```python
from build123d import *

# Parameters (mm, degrees)
ESBO_O1_R                = 1.5
RESSALTO_EXTRUS_O1_DEPTH = 1
ESBO_O2_W                = 25
ESBO_O2_H                = 1
RESSALTO_EXTRUS_O2_DEPTH = 5
ESBO_O3_R                = 1.75
CORTE_EXTRUS_O1_DEPTH    = 5
ESBO_O4_W                = 4.5
ESBO_O4_H                = 1
RESSALTO_EXTRUS_O3_DEPTH = 1.1
ESBO_O5_W                = 4.5
ESBO_O5_H                = 6.5
RESSALTO_EXTRUS_O4_DEPTH = 1


with BuildPart() as part:
    # Esboço1 → Ressalto-extrusão1 (new body)
    with BuildSketch(Plane.XY):
        Polygon((-2.930659551, 5.581459362), (-2.930659551, -2.668540638), (22.069340449, -2.668540638), (22.069340449, 5.581459362), (17.319340449, 5.581459362), (17.319340449, -1.668540638), (1.819340449, -1.668540638), (1.819340449, 5.581459362), align=None)
        with Locations((-0.180659551, 2.831459362)):
            Circle(ESBO_O1_R, mode=Mode.SUBTRACT)
        with Locations((19.319340449, 2.831459362)):
            Circle(ESBO_O1_R, mode=Mode.SUBTRACT)
    extrude(amount=RESSALTO_EXTRUS_O1_DEPTH)

    # Esboço2 → Ressalto-extrusão2 (add)
    with BuildSketch(Plane(origin=(0, 0, 0), x_dir=(-1, 0, 0), z_dir=(0, 0, -1))):
        with Locations((-9.569340449, -2.168540638)):
            Rectangle(ESBO_O2_W, ESBO_O2_H)
    extrude(amount=RESSALTO_EXTRUS_O2_DEPTH)

    # Esboço3 → Corte-extrusão1 (cut)
    with BuildSketch(Plane(origin=(0, -1.668540638, 0), x_dir=(1, 0, 0), z_dir=(0, 1, 0))):
        with Locations(Location((9.627945133, 2.5, 0), (0, 0, 180))):
            Circle(ESBO_O3_R)
    extrude(amount=-CORTE_EXTRUS_O1_DEPTH, mode=Mode.SUBTRACT)

    # Esboço4 → Ressalto-extrusão3 (add)
    with BuildSketch(Plane.XY.offset(1)):
        with Locations((-0.680659551, -0.418540638)):
            Rectangle(ESBO_O4_W, ESBO_O4_H)
        with Locations((19.819340449, -0.418540638)):
            Rectangle(ESBO_O4_W, ESBO_O4_H)
    extrude(amount=RESSALTO_EXTRUS_O3_DEPTH)

    # Esboço5 → Ressalto-extrusão4 (add)
    with BuildSketch(Plane.XY.offset(2.1)):
        with Locations((-0.680659551, 2.331459362)):
            Rectangle(ESBO_O5_W, ESBO_O5_H)
        with Locations((19.819340449, 2.331459362)):
            Rectangle(ESBO_O5_W, ESBO_O5_H)
    extrude(amount=RESSALTO_EXTRUS_O4_DEPTH)


solid = part.part
```
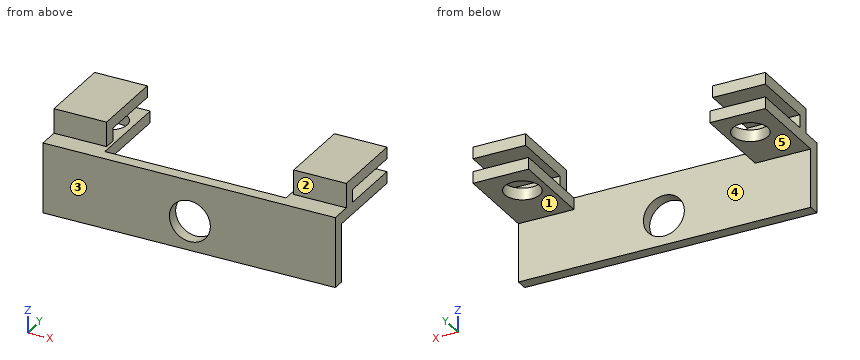
Input: part model. Units: mm. Frame: model coordinates. Face numbers are marked on the shaded views. A direction names the side the tool comes from. Give positions to 0.01 mm unless a question says otherwise; leave off trailing zeros. Write each loop counter-clockwise with the first axis right and the second up, starting at its lowest first coordinate (ties: lowest second). Pieces come first, ordered by that corner, then holes. Notation, with made-up numbers: (86.25, 75) - (98.25, 75) arc R26 ccw to (98.25, 94) - close; hole circle Ø2 at (45.5, 35.5). An arc over 180 degrees is marked (long way). Write item = value, one per line. Start each with the question number.
1) Cut plane A-A (y = 4.75). Return loops of the section in (x, z).
2) Pin query (flat end, axial travel): pin 1 (0.6 mm diameter, centred on x = 20.5, z = 1.5, fed in from +Y); pin 2 (1 mm diameter, centred on x = 21, z = 2.5, fed in from -Y); pin 3 (1.3 mm diameter, centred on x = 19, y = 4, fed in from -Z). Return the tip coordinate at first contact, or that it passes through.
3) Cut plane B-B (z = -2.5). Return loops of the section in (x, y), and give its area (3 significant figures).
4) Draft query along X for the marked faces 4 and 5. Return one class per face: pulls with the +X half, pulls with the -X half, needs draft (parallel to the pull), parting line crosses it, or undercut.
5) Material intervals for L1, parallel to Z at x = 20.75, y = 0.75; L2, parallel to X at y = 1.25, z = 0.25; L3, parallel to X at y = 2.5, z = 2.75, sorted ascending. Write a range as [from, to].
6) Cut plane D-D (x = 18.5). Return loops of the section in (y, z) (3 decimals).
7) Cut plane C-C (y = -0.25). Return loops of the section in (x, z).
8) Reachability of the marked faces 1, 2 and 3 from +Z, -Z, +X, -X, +Y, -Y: full face, straight path, thin tool, end or side. Return the list, or none.
Answers follow:
q1.outline = (-2.93, 0) - (1.82, 0) - (1.82, 1) - (-2.93, 1) - close; (-2.93, 2.1) - (1.57, 2.1) - (1.57, 3.1) - (-2.93, 3.1) - close; (17.32, 0) - (22.07, 0) - (22.07, 1) - (17.32, 1) - close; (17.57, 2.1) - (22.07, 2.1) - (22.07, 3.1) - (17.57, 3.1) - close
q2.pin_1 = 0.08
q2.pin_2 = -0.92
q2.pin_3 = 0
q3.outline = (-2.93, -2.67) - (7.88, -2.67) - (7.88, -1.67) - (-2.93, -1.67) - close; (11.38, -2.67) - (22.07, -2.67) - (22.07, -1.67) - (11.38, -1.67) - close
q3.area = 21.5 mm^2
q4.face_4 = undercut
q4.face_5 = needs draft
q5.L1 = [0, 1], [2.1, 3.1]
q5.L2 = [-2.93, 1.82], [17.32, 22.07]
q5.L3 = [-2.93, 1.57], [17.57, 22.07]
q6.outline = (-2.669, -5) - (-1.669, -5) - (-1.669, 0) - (1.575, 0) - (1.575, 1) - (0.081, 1) - (0.081, 2.1) - (5.581, 2.1) - (5.581, 3.1) - (-0.919, 3.1) - (-0.919, 1) - (-2.669, 1) - close; (4.088, 0) - (5.581, 0) - (5.581, 1) - (4.088, 1) - close
q7.outline = (-2.93, 0) - (1.82, 0) - (1.82, 1) - (1.57, 1) - (1.57, 3.1) - (-2.93, 3.1) - close; (17.32, 0) - (22.07, 0) - (22.07, 3.1) - (17.57, 3.1) - (17.57, 1) - (17.32, 1) - close
q8.face_1 = -Z, +X, -X, +Y
q8.face_2 = +Z, +X, -X, -Y
q8.face_3 = +Z, -Z, +X, -X, -Y
